from build123d import *

# Parameters (mm, degrees)
SKETCH1_R           = 4
BOSS_EXTRUDE1_DEPTH = 6.35
SKETCH2_R           = 3
CUT_EXTRUDE1_DEPTH  = 10
SKETCH3_R           = 2
CUT_EXTRUDE2_DEPTH  = 7.35
SKETCH4_R           = 2.75
CUT_EXTRUDE3_DEPTH  = 10
BOSS_EXTRUDE2_DEPTH = 6.35


with BuildPart() as part:
    # Sketch1 → Boss-Extrude1 (new body)
    with BuildSketch(Plane.XY):
        with BuildLine():
            Line((72, 134.675), (-72, 134.675))
            ThreePointArc((-72, 134.675), (-74.121320344, 133.796320344), (-75, 131.675))
            Line((-75, 131.675), (-75, -62.325))
            ThreePointArc((-75, -62.325), (-74.121320344, -64.446320344), (-72, -65.325))
            Line((-72, -65.325), (72, -65.325))
            ThreePointArc((72, -65.325), (74.121320344, -64.446320344), (75, -62.325))
            Line((75, -62.325), (75, 131.675))
            ThreePointArc((75, 131.675), (74.121320344, 133.796320344), (72, 134.675))
        make_face()
        with Locations((-65, 50.325)):
            Circle(SKETCH1_R, mode=Mode.SUBTRACT)
        with Locations((-65, -50.325)):
            Circle(SKETCH1_R, mode=Mode.SUBTRACT)
        with Locations((65, -50.325)):
            Circle(SKETCH1_R, mode=Mode.SUBTRACT)
        with Locations((65, 50.325)):
            Circle(SKETCH1_R, mode=Mode.SUBTRACT)
    extrude(amount=BOSS_EXTRUDE1_DEPTH)

    # Sketch2 → Cut-Extrude1 (cut)
    with BuildSketch(Plane.XY.offset(6.35)):
        with Locations((0, -59.325)):
            Circle(SKETCH2_R)
        with BuildLine():
            ThreePointArc((-36.53351789, 130.62609934), (-40.668585297, 129.78392163), (-44.784296659, 128.851738315))
            ThreePointArc((-44.784296659, 128.851738315), (-47.141646379, 125.021894676), (-43.31180274, 122.664544956))
            ThreePointArc((-43.31180274, 122.664544956), (-39.331414703, 123.56607837), (-35.332307043, 124.380565536))
            ThreePointArc((-35.332307043, 124.380565536), (-32.810145565, 128.103937862), (-36.53351789, 130.62609934))
        make_face()
        with BuildLine():
            ThreePointArc((-43.164725519, -58.383142339), (-43.175, -59.325), (-43.164725519, -60.266857661))
            ThreePointArc((-43.164725519, -60.266857661), (-39.921218823, -63.371839837), (-36.816236647, -60.128333141))
            ThreePointArc((-36.816236647, -60.128333141), (-36.825, -59.325), (-36.816236647, -58.521666859))
            ThreePointArc((-36.816236647, -58.521666859), (-39.921218823, -55.278160163), (-43.164725519, -58.383142339))
        make_face()
        with BuildLine():
            ThreePointArc((36.53351789, 130.62609934), (40.668585297, 129.78392163), (44.784296659, 128.851738315))
            ThreePointArc((44.784296659, 128.851738315), (47.141646379, 125.021894676), (43.31180274, 122.664544956))
            ThreePointArc((43.31180274, 122.664544956), (39.331414703, 123.56607837), (35.332307043, 124.380565536))
            ThreePointArc((35.332307043, 124.380565536), (32.810145565, 128.103937862), (36.53351789, 130.62609934))
        make_face()
        with BuildLine():
            ThreePointArc((43.164725519, -58.383142339), (43.175, -59.325), (43.164725519, -60.266857661))
            ThreePointArc((43.164725519, -60.266857661), (39.921218823, -63.371839837), (36.816236647, -60.128333141))
            ThreePointArc((36.816236647, -60.128333141), (36.825, -59.325), (36.816236647, -58.521666859))
            ThreePointArc((36.816236647, -58.521666859), (39.921218823, -55.278160163), (43.164725519, -58.383142339))
        make_face()
    extrude(amount=-CUT_EXTRUDE1_DEPTH, mode=Mode.SUBTRACT)

    # Sketch3 → Cut-Extrude2 (cut, through all)
    with BuildSketch(Plane.XY.offset(6.35)):
        with Locations((-70, 129.675)):
            Circle(SKETCH3_R)
        with Locations((-70, 119.675)):
            Circle(SKETCH3_R)
        with Locations((70, 119.675)):
            Circle(SKETCH3_R)
        with Locations((70, 129.675)):
            Circle(SKETCH3_R)
    extrude(amount=-CUT_EXTRUDE2_DEPTH, mode=Mode.SUBTRACT)

    # Sketch4 → Cut-Extrude3 (cut)
    with BuildSketch(Plane(origin=(-33.865437688, -165.327994616, 0), x_dir=(-1, 0, 0), z_dir=(0, 0, -1))):
        with Locations((-67.365437688, 232.826497308)):
            Circle(SKETCH4_R)
        with Locations((-87.365437688, 232.826497308)):
            Circle(SKETCH4_R)
        with Locations((-87.365437688, 257.826497308)):
            Circle(SKETCH4_R)
        with Locations((-67.365437688, 257.826497308)):
            Circle(SKETCH4_R)
    extrude(amount=-CUT_EXTRUDE3_DEPTH, mode=Mode.SUBTRACT)

    # Sketch5 → Boss-Extrude2 (add)
    with BuildSketch(Plane.XY.offset(6.35)):
        with BuildLine():
            Line((72, 134.675), (192, 134.675))
            Line((192, 134.675), (192, -65.325))
            Line((192, -65.325), (72, -65.325))
            ThreePointArc((72, -65.325), (74.121320344, -64.446320344), (75, -62.325))
            Line((75, -62.325), (75, 131.675))
            ThreePointArc((75, 131.675), (74.121320344, 133.796320344), (72, 134.675))
        make_face()
    extrude(amount=-BOSS_EXTRUDE2_DEPTH)


solid = part.part
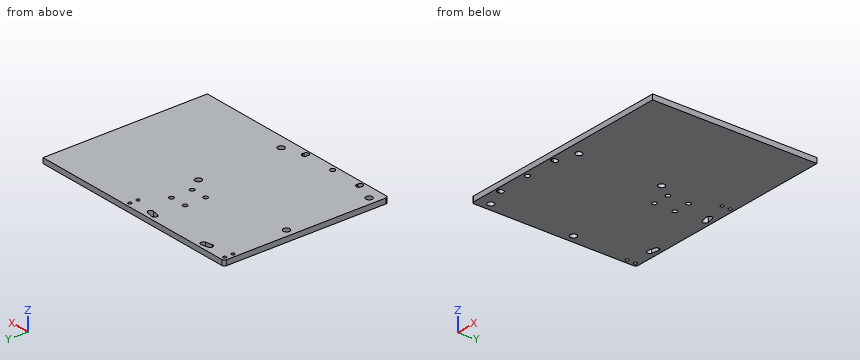
Read the model definition and answer for the solid it produces. Units are mm, in the model's axes. Coordinates: 2 decimals unless noted, no trailing zeros. Loops run counter-clockwise (first coordinate to the right, second up) from the corner with the lowest first, then second, coordinate; pieces in that order, holes last.
Q1. Consider probe 1 along Y at (x, z) = (65, 2) (3 decimals); probe 2 along Y at (x, z) = (-70, 5) (3 decimals); probe 3 along Y at (x, z) = (33.5, 4.5) (1 decimal). Determine where each line is inside the solid, lowest interval first.
Q2. The part is cut by section A-A on x = 0. Write down the section's boundary in (y, z) (3 decimals), and give its area (3 significant figures).
Q3. This flat-tipped pin is pushed along its axis until it touches: pin 1 Ø3.5 at (x, y) = (53.5, 67.5) entering from +Z. Where does it stop, or does it pass through?
Q4. The part is cut by section B-B on x = 65. Write down the section's boundary in (y, z) (3 decimals), and give its area (3 significant figures).
Results below:
1. probe 1: y = -65.325 to -54.325, -46.325 to 46.325, 54.325 to 134.675
1. probe 2: y = -65.325 to 117.675, 121.675 to 127.675, 131.675 to 134.675
1. probe 3: y = -65.3 to 64.7, 70.2 to 89.7, 95.2 to 125.5, 129.6 to 134.7
2. outline: (-65.325, 0) - (-62.325, 0) - (-62.325, 6.35) - (-65.325, 6.35) - close; (-56.325, 0) - (134.675, 0) - (134.675, 6.35) - (-56.325, 6.35) - close
2. area: 1,230 mm2
3. pin 1: passes through
4. outline: (-65.325, 0) - (-54.325, 0) - (-54.325, 6.35) - (-65.325, 6.35) - close; (-46.325, 0) - (46.325, 0) - (46.325, 6.35) - (-46.325, 6.35) - close; (54.325, 0) - (134.675, 0) - (134.675, 6.35) - (54.325, 6.35) - close
4. area: 1,170 mm2
